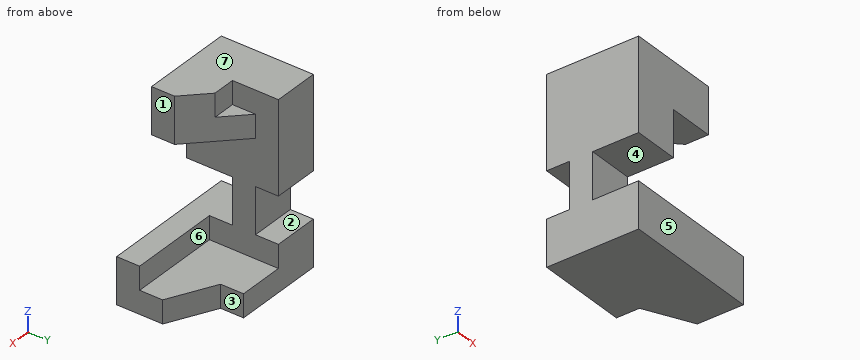
```python
from build123d import *

# Parameters (mm, degrees)
SKETCH1_W           = 6
SKETCH1_H           = 4
BOSS_EXTRUDE1_DEPTH = 8
SKETCH2_W           = 2
SKETCH2_H           = 2
CUT_EXTRUDE1_DEPTH  = 1
SKETCH4_W           = 5
SKETCH4_H           = 3
CUT_EXTRUDE13_DEPTH = 4
SKETCH5_W           = 4
SKETCH5_H           = 1
CUT_EXTRUDE14_DEPTH = 4
SKETCH6_W           = 2
SKETCH6_H           = 2
CUT_EXTRUDE15_DEPTH = 3
CUT_EXTRUDE16_DEPTH = 1
SKETCH8_W           = 1
SKETCH8_H           = 1
CUT_EXTRUDE17_DEPTH = 2
SKETCH10_W          = 2
SKETCH10_H          = 2
CUT_EXTRUDE18_DEPTH = 5
SKETCH12_W          = 2
SKETCH12_H          = 1
CUT_EXTRUDE19_DEPTH = 2
CUT_EXTRUDE20_DEPTH = 2


with BuildPart() as part:
    # Sketch1 → Boss-Extrude1 (new body)
    with BuildSketch(Plane.XY):
        Rectangle(SKETCH1_W, SKETCH1_H)
    extrude(amount=BOSS_EXTRUDE1_DEPTH)

    # Sketch2 → Cut-Extrude1 (cut)
    with BuildSketch(Plane(origin=(0, 2, 0), x_dir=(1, 0, 0), z_dir=(0, 1, 0))):
        with Locations((-2, -3)):
            Rectangle(SKETCH2_W, SKETCH2_H)
    extrude(amount=-CUT_EXTRUDE1_DEPTH, mode=Mode.SUBTRACT)

    # Sketch4 → Cut-Extrude13 (cut)
    with BuildSketch(Plane(origin=(3, 0, 0), x_dir=(0, 0, -1), z_dir=(1, 0, 0))):
        with Locations((-3.5, 0.5)):
            Rectangle(SKETCH4_W, SKETCH4_H)
    extrude(amount=-CUT_EXTRUDE13_DEPTH, mode=Mode.SUBTRACT)

    # Sketch5 → Cut-Extrude14 (cut)
    with BuildSketch(Plane(origin=(3, 0, 0), x_dir=(0, 0, -1), z_dir=(1, 0, 0))):
        with Locations((-4, -1.5)):
            Rectangle(SKETCH5_W, SKETCH5_H)
    extrude(amount=-CUT_EXTRUDE14_DEPTH, mode=Mode.SUBTRACT)

    # Sketch6 → Cut-Extrude15 (cut, through all)
    with BuildSketch(Plane(origin=(-1, 0, 0), x_dir=(0, 0, -1), z_dir=(1, 0, 0))):
        with Locations((-3, -1)):
            Rectangle(SKETCH6_W, SKETCH6_H)
    extrude(amount=-CUT_EXTRUDE15_DEPTH, mode=Mode.SUBTRACT)

    # Sketch7 → Cut-Extrude16 (cut)
    with BuildSketch(Plane(origin=(0, 0, 0), x_dir=(-1, 0, 0), z_dir=(0, 0, -1))):
        Polygon((-1, 2), (-1, 1), (-3, 0), (-3, 2), align=None)
    extrude(amount=-CUT_EXTRUDE16_DEPTH, mode=Mode.SUBTRACT)

    # Sketch8 → Cut-Extrude17 (cut)
    with BuildSketch(Plane(origin=(0, 2, 0), x_dir=(1, 0, 0), z_dir=(0, 1, 0))):
        with Locations((-0.5, -7.5)):
            Rectangle(SKETCH8_W, SKETCH8_H)
    extrude(amount=-CUT_EXTRUDE17_DEPTH, mode=Mode.SUBTRACT)

    # Sketch10 → Cut-Extrude18 (cut, through all)
    with BuildSketch(Plane(origin=(0, 2, 0), x_dir=(1, 0, 0), z_dir=(0, 1, 0))):
        with Locations((2, -7)):
            Rectangle(SKETCH10_W, SKETCH10_H)
    extrude(amount=-CUT_EXTRUDE18_DEPTH, mode=Mode.SUBTRACT)

    # Sketch12 → Cut-Extrude19 (cut)
    with BuildSketch(Plane(origin=(1, 0, 0), x_dir=(0, 0, -1), z_dir=(1, 0, 0))):
        with Locations((-7, 1.5)):
            Rectangle(SKETCH12_W, SKETCH12_H)
    extrude(amount=-CUT_EXTRUDE19_DEPTH, mode=Mode.SUBTRACT)

    # Sketch13 → Cut-Extrude20 (cut)
    with BuildSketch(Plane.XY.offset(8)):
        Polygon((1, -1), (-1, 1), (1, 1), align=None)
    extrude(amount=-CUT_EXTRUDE20_DEPTH, mode=Mode.SUBTRACT)


solid = part.part
```
Geometry: final body of the model. Coordinates: model frame, mm. Face numbers are marked on the shaded views. A direction names the side the tool comes from. Coordinates: 2 decimals unless noted, no trailing zeros. Order: outer loops, then holes, each group sorted by start corner. A loop starts at its lowest first (then second) coordinate and runs counter-clockwise, first axis right, second up. Notation, with made-up numbers: (-16, 24.5) - (10, 24.5) arc R31 ccw to (10, 56.5) - close; hole circle Ø3 at (74.25, 26.5). An arc over 180 degrees is marked (long way). Write each question's results on one line, items separated by ' | '.
1) Pull-direction query (Z, two-part tool) for the marked faces 5, 6 and 7; classes: pulls with the +Z half, pulls with the -Z half, needs draft (parallel to the pull), parting line crosses it, or undercut.
Results list:
face 5: needs draft | face 6: undercut | face 7: pulls with the +Z half
2) Line query: line 1 (Z direction, x = 0, y = -1.35); line 2 (Z direction, x = -0.95, y = 0.65); line 3 (X direction, y = 1.8, z = 4.5). Output: solid intervals per line, ascending. Write a range as from..to.
Results list:
line 1: 0..2, 6..8 | line 2: 0..1, 6..7 | line 3: -3..-1
3) Section C-C, the plane y = -1.55. Return loops of the section in (x, z).
Results list:
outline: (-3, 0) - (3, 0) - (3, 2) - (-3, 2) - close; (-3, 4) - (-1, 4) - (-1, 6) - (1, 6) - (1, 8) - (-3, 8) - close
4) Set-up query: the marked faces 1, 2, 3 and 4. Return all of +Z, -Z, +X, -X, +Y, -Y with unobstructed straight access to the full face (end or side cutting, diameter ignored); none if empty.
Results list:
face 1: +Z, +X, +Y, -Y | face 2: +X, -X, +Y | face 3: +Z, -Z, +X, +Y | face 4: +X, -X, -Y
5) Section B-B, the plane x = -0.8. Return loops of the section in (y, z).
Results list:
outline: (-2, 0) - (2, 0) - (2, 1) - (-1, 1) - (-1, 2) - (-2, 2) - close; (-2, 6) - (0.8, 6) - (0.8, 7) - (0, 7) - (0, 8) - (-2, 8) - close
6) Section A-A, the plane y = -0.35. Return loops of the section in (x, z).
Results list:
outline: (-3, 0) - (3, 0) - (3, 1) - (-1, 1) - (-1, 2) - (-3, 2) - close; (-3, 4) - (-1, 4) - (-1, 6) - (0.35, 6) - (0.35, 8) - (-3, 8) - close
7) Pin query (flat end, axial travel): pin 1 (1.1 mm diameter, centred on y = 1.5, z = 0.5, fed in from +X); pin 2 (2 mm diameter, centred on x = 1.5, y = -1.5, fed in from -Z); pin 3 (0.8 mm diameter, centred on x = 0.5, z = 1.5, fed in from +Y); pin 4 (0.8 mm diameter, centred on x = -0.5, y = 0.5, fed in from +Z). Return the tip coordinate at first contact, or that it passes through.
Results list:
pin 1: x = 1.1 | pin 2: z = 0 | pin 3: y = -1 | pin 4: z = 7
8) Section D-D, the plane x = -2.05. Return loops of the section in (y, z).
Results list:
outline: (-2, 0) - (2, 0) - (2, 2) - (1, 2) - (1, 4) - (2, 4) - (2, 8) - (-2, 8) - (-2, 4) - (0, 4) - (0, 2) - (-2, 2) - close
